Autodesk Inventor part; units mm, degrees
ref_plane "YZ Plane" through (0, 0, 0) normal (1, 0, 0) x (0, 1, 0)
ref_plane "XZ Plane" through (0, 0, 0) normal (0, 1, 0) x (-1, 0, 0)
ref_plane "XY Plane" through (0, 0, 0) normal (0, 0, 1) x (1, 0, 0)
sketch "Sketch1" plane through (0, 0, 0) normal (1, 0, 0) x (0, 1, 0)
  line L0 (0, 0) -> (-150, 0)
  line L1 (-150, 0) -> (-150, -100)
  line L2 (-150, -100) -> (0, -100)
  line L3 (0, -100) -> (0, 0)
  dimension "d0" = 150
  dimension "d1" = 100
extrude "Extrusion1" add sketch "Sketch1" along normal blind 20
sketch "Sketch2" plane through (20, 0, 0) normal (1, 0, 0) x (0, 0, -1)
  line L0 (32.1942, -72.8605) -> (72.1942, -72.8605)
  line L1 (72.1942, -72.8605) -> (72.1942, -32.8605)
  line L2 (72.1942, -32.8605) -> (32.1942, -32.8605)
  line L3 (32.1942, -32.8605) -> (32.1942, -72.8605)
  point P0 (0, 0)
  dimension "d4" = 40
  dimension "d5" = 40
extrude "Extrusion2" add sketch "Sketch2" along normal blind 40
sketch "Sketch3" plane through (60, 0, 0) normal (1, 0, 0) x (0, 0, -1)
  line L0 (32.1942, -72.8605) -> (32.1942, -32.8605)
  line L1 (32.1942, -72.8605) -> (32.1942, -32.8605)
  line L2 (32.1942, -32.8605) -> (32.1942, -52.8605)
  line L3 (48.2142, -59.6131) -> (57.4566, -59.6131)
  line L4 (57.4566, -59.6131) -> (57.4566, -46.3658)
  line L5 (57.4566, -46.3658) -> (48.2142, -46.3658)
  line L6 (48.2142, -46.3658) -> (48.2142, -59.6131)
  point P0 (0, 0)
extrude "Extrusion3" add sketch "Sketch3" along normal blind 15
sketch "Sketch4" plane through (60, 0, 0) normal (1, 0, 0) x (0, 0, -1)
  point P0 (0, 0)
sketch "Sketch5" plane through (60, 0, 0) normal (1, 0, 0) x (0, 0, -1)
  line L0 (57.1037, -71.8566) -> (71.8566, -60.4104)
  line L1 (71.8566, -60.4104) -> (45.9119, -32.8605)
  line L2 (32.1942, -32.8605) -> (72.1942, -32.8605)
  line L3 (33.6968, -44.3638) -> (57.1037, -71.8566)
  line L4 (32.1942, -42.5989) -> (45.9119, -32.8605)
  line L5 (32.1942, -42.5989) -> (57.1037, -71.8566)
  point P0 (0, 0)
extrude "Extrusion4" add sketch "Sketch5" along normal blind 10
sketch "Sketch6" plane through (60, -42.5989, -32.1942) normal (0, 0.8154167, 0.5788745) x (1, 0, 0)
  line L0 (0, 16.823) -> (10, 16.823)
  line L1 (0, 0) -> (10, 0)
  line L2 (10, 16.823) -> (0, 16.823)
  line L3 (0, 16.823) -> (0, 0)
  line L4 (0, 0) -> (10, 0)
  line L5 (10, 0) -> (10, 16.823)
  point P0 (-60, -1.5923)
extrude "Extrusion5" add sketch "Sketch6" along normal blind 200
sketch "Sketch7" plane through (60, -42.5989, -32.1942) normal (0, -0.5788745, 0.8154167) x (1, 0, 0)
  line L0 (10, 0) -> (10, 200)
  line L1 (0, 0) -> (0, 200)
  line L2 (10, 200) -> (0, 200)
  line L3 (0, 200) -> (0, 182.714)
  line L4 (0, 182.714) -> (10, 182.714)
  line L5 (10, 182.714) -> (10, 200)
  point P0 (-60, 53.3722)
extrude "Extrusion6" add sketch "Sketch7" along normal blind 300
sketch "Sketch8" plane through (70, 0, 0) normal (1, 0, 0) x (0, 0, -1)
  point P0 (0, 0)
sketch "Sketch9" plane through (70, 0, 0) normal (1, 0, 0) x (0, 0, -1)
  circle A0 centre (-71.8205, 116.6834) radius 6.7198
  point P0 (0, 0)
extrude "Extrusion7" cut sketch "Sketch9" along normal through all both and the other way through all
sketch "Sketch10" plane through (70, 0, 0) normal (1, 0, 0) x (0, 0, -1)
  point P0 (0, 0)
sketch "Sketch11" plane through (70, 0, 0) normal (1, 0, 0) x (0, 0, -1)
  circle A0 centre (-318.1993, -56.6737) radius 3.8597
  point P0 (0, 0)
extrude "Extrusion8" cut sketch "Sketch11" along normal through all both and the other way through all
sketch "Sketch16" plane through (20, 0, 0) normal (1, 0, 0) x (0, 0, -1)
  point P0 (0, 0)
sketch "Sketch17" plane through (20, 0, 0) normal (1, 0, 0) x (0, 0, -1)
  line L0 (32.6643, -74.5991) -> (72.9814, -74.5991)
  line L1 (72.9814, -74.5991) -> (72.9814, -77.9588)
  line L2 (72.9814, -77.9588) -> (32.6643, -77.9588)
  line L3 (32.6643, -77.9588) -> (32.6643, -74.5991)
  point P0 (0, 0)
extrude "Extrusion9" add sketch "Sketch17" along normal blind 40
sketch "Sketch18" plane through (20, -77.9588, -72.9814) normal (0, -1, 0) x (1, 0, 0)
  line L0 (0, 0.7872) -> (40, 0.7872)
  line L1 (40, 40.3171) -> (40, 0.7872)
  line L2 (40, 0.7872) -> (0, 0.7872)
  line L3 (0, 0.7872) -> (0, 40.3171)
  line L4 (0, 40.3171) -> (40, 40.3171)
  line L5 (40, 40.3171) -> (40, 0)
  line L6 (40, 20.1585) -> (0, 20.5522)
  line L7 (20, 40.3171) -> (20, 0)
  line L8 (0, 0) -> (40, 0)
  line L9 (40, 40.3171) -> (20, 40.3171)
  line L10 (30, 40.3171) -> (20, 40.3171)
  line L11 (0, 40.3171) -> (40, 40.3171)
  line L12 (0, 40.3171) -> (20, 40.3171)
  circle A0 centre (30, 30.5773) radius 1.5
  circle A1 centre (30, 11.3652) radius 1.5
  circle A2 centre (8.8768, 11.3652) radius 1.5
  circle A3 centre (8.8768, 30.5773) radius 1.5
  point P0 (-20, 72.9814)
  dimension "d22" = 3
  dimension "d23" = 3
  dimension "d24" = 3
  dimension "d25" = 3
extrude "Extrusion10" cut sketch "Sketch18" along normal through all both and the other way through all contours A0 | A1 | A2 | A3
properties part number "horizontal"
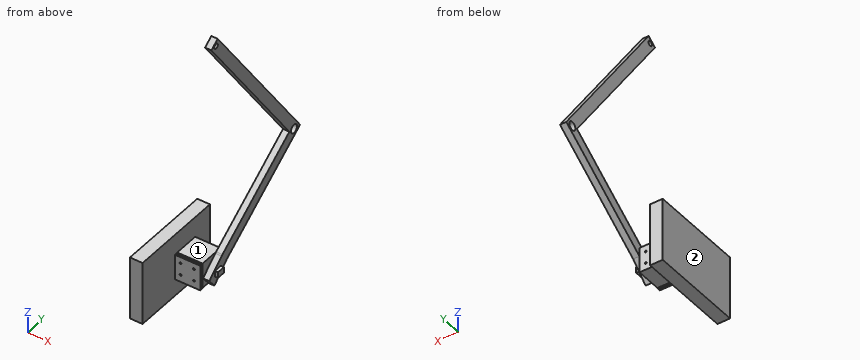
Work out the finished part from the listing and answer in its coordinate system (mm). Face numbers are marked on the shaded views. Round coordinates to 2 decimals unless told otherwise and drop trailing zeros. Loops run counter-clockwise (first coordinate to the right, second up) from the corner with the lowest first, then second, coordinate; pieces in that order, holes last. Notation, with made-up numbers: (27.5, 42.5) -> (78.5, 42.5) arc R17 cw to (78.5, 73.5) -> close; hole circle Ø3 at (27.25, -2). An arc over 180 degrees is marked (long way). Write each question's results on one line, items separated by ' | '. Start each with the question number.
1. Section D-D (y = -89.5) is taken. Determine the outline of the cut face in (x, z).
2. Section B-B (y = 55) is taken. Determine the outline of the cut face in (x, z).
3. Section C-C (x = 13.5) is taken. Determine the outline of the cut face in (y, z), plus the area to 3 significant figures.
4. Section A-A (x = 39) is taken. Determine the outline of the cut face in (y, z).
5. Find the intervals of material crossed by probe 1 along Z at (x, y) = (50, -59); probe 2 along Z at (x, y) = (61, 59.5); probe 3 along X at (y, z) = (-25, 269), in increasing order. Write a range as from..to.
6. For a pull along X with two mould halves and no side action, classify the marked faces 1 and 2 as +X half, -X half, draft (parallel to the pull), parting line (faces both ways), or undercut.
7. Given pin 1 Ø5.5 at (x, z) = (72, -52.5) entering from +Y; pin 2 Ø22 at (x, z) = (5.5, -47.5) entering from +Y; pin 3 Ø10 at (x, y) = (58, 19) entering from -Z, each flat-ended and moving along its own axis, determine where each tip first touches the part or whether it passes through.
Evaluation:
1) outline: (0, -100) -> (20, -100) -> (20, 0) -> (0, 0) -> close
2) outline: (60, 16.46) -> (70, 16.46) -> (70, 37.09) -> (60, 37.09) -> close; (60, 145.96) -> (70, 145.96) -> (70, 175.82) -> (60, 175.82) -> close
3) outline: (-150, -100) -> (0, -100) -> (0, 0) -> (-150, 0) -> close | area: 15,000 mm2
4) outline: (-77.96, -72.98) -> (-74.6, -72.98) -> (-74.6, -32.66) -> (-77.96, -32.66) -> close; (-72.86, -72.19) -> (-32.86, -72.19) -> (-32.86, -32.19) -> (-72.86, -32.19) -> close
5) probe 1: z = -72.19..-63.12, -60.12..-43.9, -40.9..-32.19 | probe 2: z = 19.66..40.29, 139.62..169.48 | probe 3: x = 60..70
6) face 1: undercut | face 2: -X half
7) pin 1: stops at y = -37.85 | pin 2: stops at y = 0 | pin 3: stops at z = -12.35
